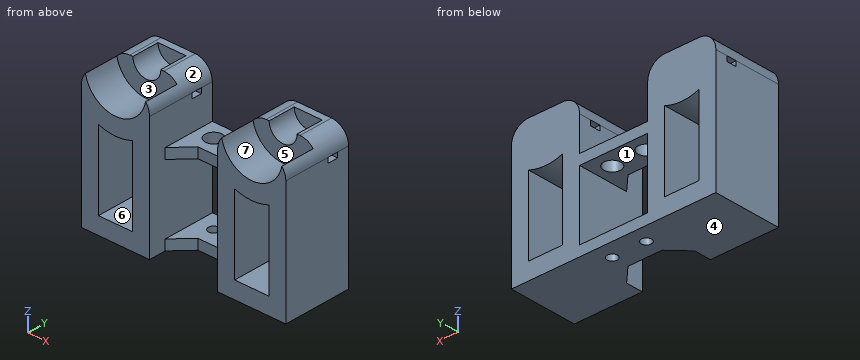
from build123d import *

# Parameters (mm, degrees)
F1_DEPTH  = 10
F2_W      = 14.1
F2_H      = 2
F3_DEPTH  = 10
F2_W_2    = 20
F5_DEPTH  = 10
F7_DEPTH  = 25
F8_W      = 3
F8_H      = 1.5
F9_DEPTH  = 100
F10_R     = 4.99999
F10_2_R   = 4.99999
F11_W     = 20
F11_H     = 3
F12_DEPTH = 10
F13_R     = 1.5
F14_DEPTH = 50
F15_R     = 2.5
F15_R_2   = 1.5
F16_DEPTH = 10
F17_SIZE  = 5


# Not quite as in the source:
# - a fillet or chamfer is up to 0.001 mm smaller than in the source, because OpenCascade refuses the exact size


with BuildPart() as f1:
    # F0 (on Front) → F1 (new body)
    with BuildSketch(Plane.XZ):
        with BuildLine():
            ThreePointArc((7, 0), (0, -7), (-7, 0))
            Line((-7, 0), (-10, 0))
            Line((-10, 0), (-10, -41))
            Line((-10, -41), (10, -41))
            Line((10, -41), (10, 0))
            Line((10, 0), (7, 0))
        make_face()
        with BuildLine():
            ThreePointArc((4.1, 0), (0, -4.1), (-4.1, 0))
            Line((-4.1, 0), (-7, 0))
            ThreePointArc((-7, 0), (0, -7), (7, 0))
            Line((7, 0), (4.1, 0))
        make_face()
    extrude(amount=F1_DEPTH)

    # F2 (on face) → F3 (join)
    with BuildSketch(Plane.XY):
        with Locations((2.95, -1)):
            Rectangle(F2_W, F2_H)
    extrude(amount=-F3_DEPTH)

    # F4 (on face) → F5 (join)
    with BuildSketch(Plane.XZ.offset(10)):
        with BuildLine():
            Line((10, 0), (9, 0))
            ThreePointArc((9, 0), (0, -9), (-9, 0))
            Line((-9, 0), (-10, 0))
            Line((-10, 0), (-10, -41))
            Line((-10, -41), (10, -41))
            Line((10, -41), (10, 0))
        make_face()
    extrude(amount=F5_DEPTH)


with BuildPart() as f1b:
    # F0 (on Front) → F1, piece 2 (new body)
    with BuildSketch(Plane.XZ):
        with BuildLine():
            Line((50, 0), (47, 0))
            ThreePointArc((47, 0), (40, -7), (33, 0))
            Line((33, 0), (30, 0))
            Line((30, 0), (30, -41))
            Line((30, -41), (50, -41))
            Line((50, -41), (50, 0))
        make_face()
        with BuildLine():
            ThreePointArc((33, 0), (40, -7), (47, 0))
            Line((47, 0), (44.1, 0))
            ThreePointArc((44.1, 0), (40, -4.1), (35.9, 0))
            Line((35.9, 0), (33, 0))
        make_face()
    extrude(amount=F1_DEPTH)

    # F2 (on face) → F3, piece 2 (join)
    with BuildSketch(Plane.XY):
        with Locations((40, -1)):
            Rectangle(F2_W_2, F2_H)
    extrude(amount=-F3_DEPTH)

    # F4 (on face) → F5, piece 2 (join)
    with BuildSketch(Plane.XZ.offset(10)):
        with BuildLine():
            Line((31, 0), (30, 0))
            Line((30, 0), (30, -41))
            Line((30, -41), (50, -41))
            Line((50, -41), (50, 0))
            Line((50, 0), (49, 0))
            ThreePointArc((49, 0), (40, -9), (31, 0))
        make_face()
    extrude(amount=F5_DEPTH)


with BuildPart() as f7_tool:
    # F6 (on face) → F7 (new body)
    with BuildSketch(Plane.XZ.offset(20)):
        with BuildLine():
            Line((5, -36), (5, -13.0766968306))
            ThreePointArc((5, -13.0766968306), (0, -14), (-5, -13.0766968306))
            Line((-5, -13.0766968306), (-5, -36))
            Line((-5, -36), (5, -36))
        make_face()
        with BuildLine():
            Line((45, -36), (45, -13.0766968306))
            ThreePointArc((45, -13.0766968306), (40, -14), (35, -13.0766968306))
            Line((35, -13.0766968306), (35, -36))
            Line((35, -36), (45, -36))
        make_face()
    extrude(amount=-F7_DEPTH)


with BuildPart() as f1_1:
    add(f1.part)

    # F7: cut by f7_tool
    add(f7_tool.part, mode=Mode.SUBTRACT)


with BuildPart() as f1b_1:
    add(f1b.part)

    # F7: cut by f7_tool
    add(f7_tool.part, mode=Mode.SUBTRACT)


with BuildPart() as f9_tool:
    # F8 (on face) → F9 (new body)
    with BuildSketch(Plane.YZ.offset(50)):
        with Locations((-5, -5.75)):
            Rectangle(F8_W, F8_H)
    extrude(amount=-F9_DEPTH)


with BuildPart() as f1_2:
    add(f1_1.part)

    # F9: cut by f9_tool
    add(f9_tool.part, mode=Mode.SUBTRACT)

    # F10#2 (radius 5 in the source; OpenCascade refuses exactly that, so slightly less here)
    f10_2_edges = [f1_2.edges().sort_by_distance(p)[0] for p in [
        (-10, -10, 0),
        (10, -10, 0),
    ]]
    fillet(f10_2_edges, radius=F10_2_R)



with BuildPart() as f1b_2:
    add(f1b_1.part)

    # F9: cut by f9_tool
    add(f9_tool.part, mode=Mode.SUBTRACT)

    # F10 (radius 5 in the source; OpenCascade refuses exactly that, so slightly less here)
    f10_edges = [f1b_2.edges().sort_by_distance(p)[0] for p in [
        (30, -10, 0),
        (50, -10, 0),
    ]]
    fillet(f10_edges, radius=F10_R)


with BuildPart() as f1_3:
    add(f1_2.part)

    add(f1b_2.part)  # F12 merges F1b
    # F11 (on face) → F12 (join)
    with BuildSketch(Plane(origin=(0, 0, 0), x_dir=(-1, 0, 0), z_dir=(0, 1, 0))):
        with Locations((-20, -39.5)):
            Rectangle(F11_W, F11_H)
        with Locations((-20, -16.5)):
            Rectangle(F11_W, F11_H)
    extrude(amount=-F12_DEPTH)

    # F13 (on face) → F14 (cut)
    with BuildSketch(Plane(origin=(0, 0, -41), x_dir=(1, 0, 0), z_dir=(0, 0, -1))):
        with Locations((15, 5)):
            Circle(F13_R)
        with Locations((25, 5)):
            Circle(F13_R)
    extrude(amount=-F14_DEPTH, mode=Mode.SUBTRACT)

    # F15 (on face) → F16 (cut)
    with BuildSketch(Plane.XY.offset(-15)):
        with Locations((15, -5)):
            Circle(F15_R)
        with Locations((15, -5)):
            Circle(F15_R_2, mode=Mode.SUBTRACT)
        with Locations((25, -5)):
            Circle(F15_R)
        with Locations((25, -5)):
            Circle(F15_R_2, mode=Mode.SUBTRACT)
    extrude(amount=-F16_DEPTH, mode=Mode.SUBTRACT)

    # F17
    f17_edges = [f1_3.edges().sort_by_distance(p)[0] for p in [
        (30, -10, -39.5),
        (10, -10, -39.5),
        (30, -10, -16.5),
        (10, -10, -16.5),
    ]]
    chamfer(f17_edges, length=F17_SIZE)


solid = f1_3.part
Check sheet for the modelled part. Datum: model origin and axes. Units: mm. Face numbers are marked on the shaded views. A direction names the side the tool comes from. Give positions to 0.01 mm unless a question says otherwise; leave off trailing zeros. Loops run counter-clockwise (first coordinate to the right, second up) from the corner with the lowest first, then second, coordinate; pieces in that order, holes last. Notation, with made-up numbers: M 74.25,-26 L 79.25,-26 A25 ccw 79.25,-1 Z; hole C -2.5,-40 d1. An arc over 180 degrees is marked long. Return JSON: item names as keys, results as strings. Group by question number.
1. Cross-section at A-A on x = 0. Record the boundary of the cut face in (y, z).
2. Cross-section at D-D on z = -23. Record the boundary of the cut face in (x, y), plus the area to 3 significant figures.
3. Thickness scan on L1, parallel to X at y = -5, z = -39.1; L2, parallel to X at y = -18, z = -35; L3, parallel to Y at x = 25, z = -15.55. Record the ranges inside material, lowest first.
4. Tool access check on the marked faces 1, 2, 3 and 4. Record the directions out of +Z, -Z, +X, -X, +Y, -Y that give a thin tool (end or side, any length) a straight path to the whole face; none if there is none.
5. Cross-section at B-B on z = -17. Record the boundary of the cut face in (x, y).
6. Go/stop test with flat-tipped pins: pin 1 (10 mm diameter, centred on x = 18, y = -6.5, fed in from +Z); pin 2 (2.5 mm diameter, centred on x = 39.5, z = -5.5, fed in from -Y); pin 3 (2 mm diameter, centred on x = 1.5, z = -2, fed in from -Y). Record where each tip stops, or that it passes through.
7. Mould release check, pull along Z, two halves, no side actions. Record for the marked faces 5, 6 and 7: released by +Z, released by -Z, zero draft, split by the parting line, or undercut.
8. Cross-section at C-C on y = -13.5. State how many separate pieces and enclosed holes the cut face has, plus the area to 3 significant figures.
Return value:
{
 "1": {"outline": "M -20,-41 L 0,-41 L 0,-36 L -20,-36 Z; M -20,-14 L 0,-14 L 0,0 L -2,0 L -2,-4.1 L -10,-4.1 L -10,-9 L -20,-9 Z; hole M -6.5,-6.5 L -3.5,-6.5 L -3.5,-5 L -6.5,-5 Z"},
 "2": {"outline": "M -10,-20 L -5,-20 L -5,0 L -10,0 Z; M 5,-20 L 10,-20 L 10,0 L 5,0 Z; M 30,-20 L 35,-20 L 35,0 L 30,0 Z; M 45,-20 L 50,-20 L 50,0 L 45,0 Z", "area": "400 mm^2"},
 "3": {"L1": "-10 to 13.5, 16.5 to 23.5, 26.5 to 50", "L2": "-10 to -5, 5 to 10, 30 to 35, 45 to 50", "L3": "-10 to -7.5, -2.5 to 0"},
 "4": {"face 1": "+Y, -Y", "face 2": "+Z, +Y, -Y", "face 3": "+Z, -Y", "face 4": "-Z, +X, -X, +Y, -Y"},
 "5": {"outline": "M -10,-20 L -5,-20 L -5,0 L -10,0 Z; M 5,-20 L 10,-20 L 10,-15 L 15,-10 L 25,-10 L 30,-15 L 30,-20 L 35,-20 L 35,0 L 5,0 Z; M 45,-20 L 50,-20 L 50,0 L 45,0 Z; hole C 15,-5 d5; hole C 25,-5 d5"},
 "6": {"pin 1": "z = -15", "pin 2": "y = -10", "pin 3": "y = -2"},
 "7": {"face 5": "zero draft", "face 6": "undercut", "face 7": "released by +Z"},
 "8": {"separate pieces": "2", "enclosed holes": "2", "area": "945 mm^2"}
}
